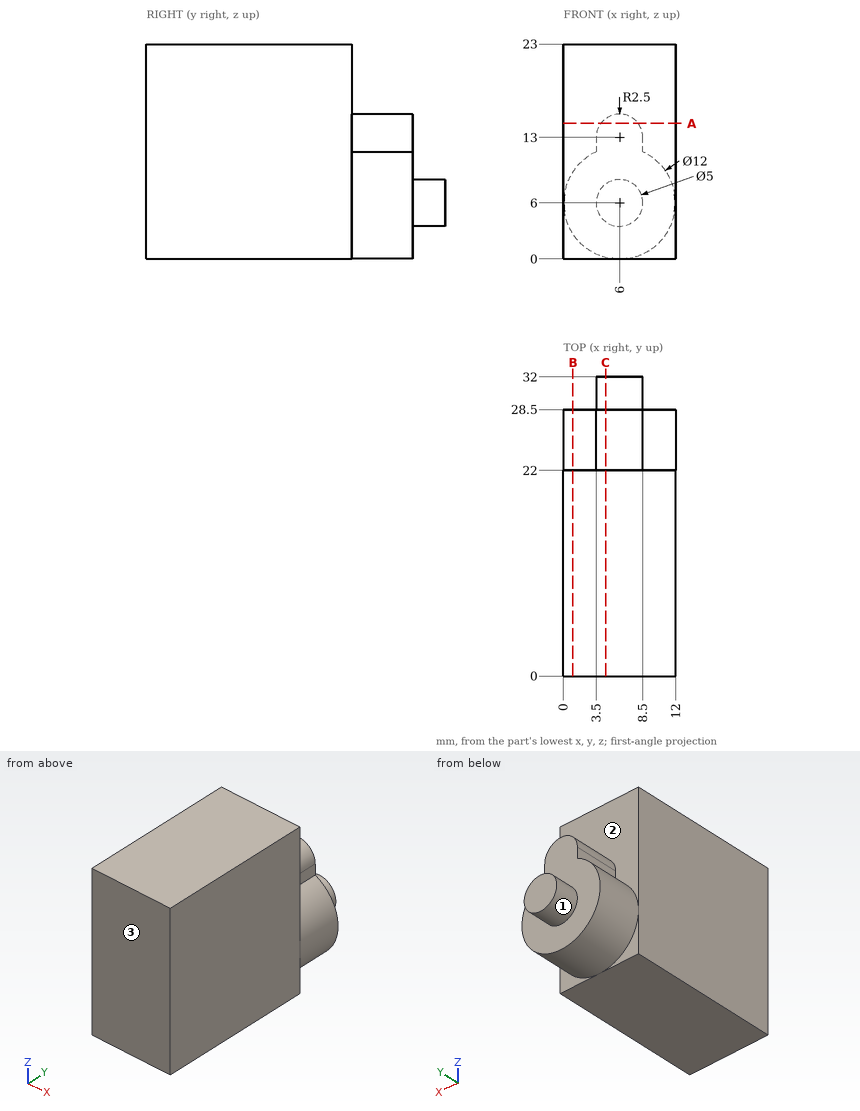
Here's the drawing with two shaded views (mm, measured from the low corner). I have some questions. A direction names the side the tool comes from. Give positions to 0.01 mm unless a question says otherwise; leave off trailing zeros. Loops run counter-clockwise (first coordinate to the right, second up) from the corner with the lowest first, then second, coordinate; pieces in that order, holes last. Notation, with made-up numbers: (40, 58.5) - (66, 58.5) arc R17 cw to (66, 88.5) - close; hole circle Ø6 at (3, 83). An arc over 180 degrees is marked (long way). Answer in a Markdown table with one row per item. Add a question column.
Q1. Which directions (+Z, -Z, +X, -X, +Y, -Y) give clear straight access to the entire face, cutting with the end or side of a thin tool? Please do the marked faces 1, 2 and 3.
Q2. Please list where these lines run through material, in increasing order: L1, parallel to Y at x = 7.75, z = 9.5; L2, parallel to Y at x = 1, z = 10.75; L3, parallel to Z at x = 9, y = 23. Write a range as from..to.
Q3. If we section it at B-B (x = 1): List the corners of the cut face in (y, z) for me.
Q4. For pin 1 (2 mm diameter, centred on x = 9, y = 27.5, fed in from -Z); pin 2 (0.8 mm diameter, centred on y = 24, z = 12, fed in from -X); pin 3 (1.8 mm diameter, centred on x = 1.5, z = 3.5, fed in from +Y); pin 4 (10 mm diameter, centred on y = 27, z = 3, fed in from +X), each with a flat end and sliding along its axis, tell me the tip position at first contact or that it passes through.
Q5. If we section it at C-C (x = 4.5): List the corners of the cut face in (y, z) for me.
Q6. If we section it at A-A (z = 14.5): List the corners of the cut face in (x, y) for me.
The answers:
| question | item | result |
|---|---|---|
| 1 | face 1 | +Y |
| 1 | face 2 | +Z, +Y |
| 1 | face 3 | +Z, -Z, +X, -X, -Y |
| 2 | L1 | y = 0..28.5 |
| 2 | L2 | y = 0..22 |
| 2 | L3 | z = 0.8..11.2 |
| 3 | outline | (0, 0) - (22, 0) - (22, 2.68) - (28.5, 2.68) - (28.5, 9.32) - (22, 9.32) - (22, 23) - (0, 23) - close |
| 4 | pin 1 | stops at z = 0.34 |
| 4 | pin 2 | stops at x = 3.5 |
| 4 | pin 3 | stops at y = 28.5 |
| 4 | pin 4 | stops at x = 12 |
| 5 | outline | (0, 0) - (22, 0) - (22, 0.19) - (28.5, 0.19) - (28.5, 4) - (32, 4) - (32, 8) - (28.5, 8) - (28.5, 15) - (22, 15) - (22, 23) - (0, 23) - close |
| 6 | outline | (0, 0) - (12, 0) - (12, 22) - (8, 22) - (8, 28.5) - (4, 28.5) - (4, 22) - (0, 22) - close |
